The model under review builds one solid part; all positions refer to its coordinate system, in mm. Coordinates: 2 decimals unless noted, no trailing zeros. Order: outer loops, then holes, each group sorted by start corner. A loop starts at its lowest first (then second) coordinate and runs counter-clockwise, first axis right, second up. Notation, with made-up numbers: M -29,39 L 21,39 A28 ccw 21,72 Z; hole C 81.25,52 d6. An arc over 180 degrees is marked long. One line per item, written item: value.
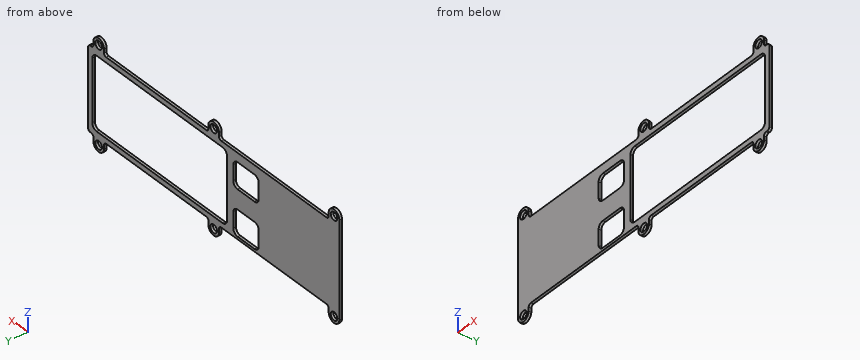
Autodesk Inventor part; units mm, degrees
ref_plane "YZ Plane" through (0, 0, 0) normal (1, 0, 0) x (0, 1, 0)
ref_plane "XZ Plane" through (0, 0, 0) normal (0, 1, 0) x (-1, 0, 0)
ref_plane "XY Plane" through (0, 0, 0) normal (0, 0, 1) x (1, 0, 0)
sketch "Sketch1" plane through (0, 0, 0) normal (0, 1, 0) x (-1, 0, 0)
  line L0 (0, 0) -> (37, 0) construction
  line L1 (37, 0) -> (37, -30) construction
  line L2 (37, -30) -> (0, -30) construction
  line L3 (0, -30) -> (0, 0) construction
  line L4 (75.5, -6) -> (38, -6) construction
  line L5 (38, -6) -> (38, -24) construction
  line L6 (38, -24) -> (75.5, -24) construction
  line L7 (75.5, -24) -> (75.5, -6) construction
  line L8 (94, 0) -> (76.5, 0) construction
  line L9 (76.5, 0) -> (76.5, -28) construction
  line L10 (76.5, -28) -> (94, -28) construction
  line L11 (94, -28) -> (94, 0) construction
  line L12 (-1, 1) -> (117.5, 1)
  line L13 (117.5, 1) -> (117.5, -31)
  line L14 (117.5, -31) -> (-1, -31)
  line L15 (-1, -31) -> (-1, 1)
  line L16 (0, 0) -> (94, 0)
  line L17 (94, 0) -> (94, -30)
  line L18 (94, -30) -> (0, -30)
  line L19 (0, -30) -> (0, 0)
  line L20 (38, -8) -> (37, -8)
  line L21 (37, -8) -> (37, -22)
  line L22 (37, -22) -> (38, -22)
  line L23 (38, -22) -> (38, -8)
  line L24 (73.5, -6) -> (40, -6)
  line L25 (40, -6) -> (40, -5)
  line L26 (40, -5) -> (73.5, -5)
  line L27 (73.5, -5) -> (73.5, -6)
  line L28 (73.5, -24) -> (40, -24)
  line L29 (40, -24) -> (40, -25)
  line L30 (40, -25) -> (73.5, -25)
  line L31 (73.5, -25) -> (73.5, -24)
  line L32 (76.5, -8) -> (75.5, -8)
  line L33 (75.5, -8) -> (75.5, -22)
  line L34 (75.5, -22) -> (76.5, -22)
  line L35 (76.5, -22) -> (76.5, -8)
  line L36 (115, -31) -> (115, -33.5) construction
  line L37 (58.25, -31) -> (58.25, -33.5) construction
  line L38 (4, -31) -> (4, -33.5) construction
  line L39 (115, 1) -> (115, 3.5) construction
  line L40 (58.25, 1) -> (58.25, 3.5) construction
  line L41 (4, 1) -> (4, 3.5) construction
  circle A0 centre (115, -33.5) radius 2.5
  circle A1 centre (58.25, -33.5) radius 2.5
  circle A2 centre (4, -33.5) radius 2.5
  circle A3 centre (4, 3.5) radius 2.5
  circle A4 centre (58.25, 3.5) radius 2.5
  circle A5 centre (115, 3.5) radius 2.5
  line L42 (117.5, 1) -> (117.5, 3.5)
  line L43 (112.5, 3.5) -> (112.5, 1)
  line L44 (60.75, 3.5) -> (60.75, 1)
  line L45 (55.75, 3.5) -> (55.75, 1)
  line L46 (6.5, 3.5) -> (6.5, 1)
  line L47 (1.5, 3.5) -> (1.5, 1)
  line L48 (1.5, -33.5) -> (1.5, -31)
  line L49 (6.5, -33.5) -> (6.5, -31)
  line L50 (55.75, -33.5) -> (55.75, -31)
  line L51 (60.75, -33.5) -> (60.75, -31)
  line L52 (117.5, -33.5) -> (117.5, -31)
  line L53 (112.5, -33.5) -> (112.5, -31)
  circle A6 centre (115, -33.5) radius 1.55
  circle A7 centre (58.25, -33.5) radius 1.55
  circle A8 centre (4, -33.5) radius 1.55
  circle A9 centre (4, 3.5) radius 1.55
  circle A10 centre (58.25, 3.5) radius 1.55
  circle A11 centre (115, 3.5) radius 1.55
  line L54 (57.75, -30) -> (58.75, -30)
  line L55 (58.75, -30) -> (58.75, -25)
  line L56 (58.75, -25) -> (57.75, -25)
  line L57 (57.75, -25) -> (57.75, -30)
  line L58 (57.75, -5) -> (58.75, -5)
  line L59 (58.75, -5) -> (58.75, 0)
  line L60 (58.75, 0) -> (57.75, 0)
  line L61 (57.75, 0) -> (57.75, -5)
  line L62 (40, -25) -> (41, -25)
  line L63 (41, -25) -> (41, -30)
  line L64 (41, -30) -> (40, -30)
  line L65 (40, -30) -> (40, -25)
  line L66 (40, -5) -> (41, -5)
  line L67 (41, -5) -> (41, 0)
  line L68 (41, 0) -> (40, 0)
  line L69 (40, 0) -> (40, -5)
  line L70 (73.5, -5) -> (72.5, -5)
  line L71 (72.5, -5) -> (72.5, 0)
  line L72 (72.5, 0) -> (73.5, 0)
  line L73 (73.5, 0) -> (73.5, -5)
  line L74 (73.5, -25) -> (72.5, -25)
  line L75 (72.5, -25) -> (72.5, -30)
  line L76 (72.5, -30) -> (73.5, -30)
  line L77 (73.5, -30) -> (73.5, -25)
  dimension "d0" = 37
  dimension "d1" = 30
  dimension "d2" = 18
  dimension "d3" = 37.5
  dimension "d4" = 1
  dimension "d5" = 6
  dimension "d6" = 17.5
  dimension "d7" = 28
  dimension "d8" = 1
  dimension "d9" = 1
  dimension "d10" = 1
  dimension "d11" = 1
  dimension "d12" = 117.5
  dimension "d13" = 2
  dimension "d14" = 2
  dimension "d15" = 1
  dimension "d16" = 1
  dimension "d17" = 2
  dimension "d18" = 2
  dimension "d19" = 2
  dimension "d20" = 2
  dimension "d21" = 2.5
  dimension "d22" = 2.5
  dimension "d23" = 5
  dimension "d24" = 2.5
  dimension "d25" = 2.5
  dimension "d26" = 2.5
  dimension "d27" = 2.5
  dimension "d28" = 5
  dimension "d29" = 5
  dimension "d30" = 2.5
  dimension "d31" = 3.1
  dimension "d32" = 3.1
  dimension "d33" = 3.1
  dimension "d34" = 3.1
  dimension "d35" = 3.1
  dimension "d36" = 3.1
  dimension "d44" = 1
  dimension "d45" = 1
  dimension "d46" = 0.5
  dimension "d47" = 0
  dimension "d48" = 1
  dimension "d49" = 1
  dimension "d50" = 1
  dimension "d51" = 1
extrude "Extrusion1" add sketch "Sketch1" along normal blind 7 contours L12 L13 L14 L15 | L47 A3 L12 | A3 L46 L12 | A3 | L14 A2 L48 | L14 L49 A2 | A2 | L45 A4 L12 | A4 L44 L12 | A4 | L14 A1 L50 | L14 L51 A1 | A1 | L43 A5 L12 | A5 L42 L12 | A5 | L14 A0 L53 | L14 L52 A0 | A0 | L16 L67 L26 L69 | L26 L27 L24 L25 | L65 L30 L63 L18 | L16 L59 L26 L61 | L29 L28 L31 L30 | L57 L30 L55 L18 | L16 L73 L26 L71 | L75 L30 L77 L18 | L23 L22 L21 L20 | L35 L34 L33 L32
sketch "Sketch2" plane through (0, 0, 0) normal (0, -1, 0) x (1, 0, 0)
  line L0 (-117.5, -33.5) -> (-117.5, 3.5)
  arc A0 (-117.5, -33.5) -> (-112.5, -33.5) centre (-115, -33.5) ccw
  line L1 (-112.5, -31) -> (-112.5, -33.5)
  line L2 (-60.75, -31) -> (-112.5, -31)
  line L3 (-60.75, -33.5) -> (-60.75, -31)
  arc A1 (-60.75, -33.5) -> (-55.75, -33.5) centre (-58.25, -33.5) ccw
  line L4 (-55.75, -31) -> (-55.75, -33.5)
  line L5 (-6.5, -31) -> (-55.75, -31)
  line L6 (-6.5, -33.5) -> (-6.5, -31)
  arc A2 (-6.5, -33.5) -> (-1.5, -33.5) centre (-4, -33.5) ccw
  line L7 (-1.5, -31) -> (-1.5, -33.5)
  line L8 (1, -31) -> (-1.5, -31)
  line L9 (1, 1) -> (1, -31)
  line L10 (-1.5, 1) -> (1, 1)
  line L11 (-1.5, 3.5) -> (-1.5, 1)
  arc A3 (-1.5, 3.5) -> (-6.5, 3.5) centre (-4, 3.5) ccw
  line L12 (-6.5, 1) -> (-6.5, 3.5)
  line L13 (-55.75, 1) -> (-6.5, 1)
  line L14 (-55.75, 3.5) -> (-55.75, 1)
  arc A4 (-55.75, 3.5) -> (-60.75, 3.5) centre (-58.25, 3.5) ccw
  line L15 (-60.75, 1) -> (-60.75, 3.5)
  line L16 (-112.5, 1) -> (-60.75, 1)
  line L17 (-112.5, 3.5) -> (-112.5, 1)
  arc A5 (-112.5, 3.5) -> (-117.5, 3.5) centre (-115, 3.5) ccw
  circle A6 centre (-58.25, 3.5) radius 1.55
  circle A7 centre (-4, 3.5) radius 1.55
  circle A8 centre (-4, -33.5) radius 1.55
  circle A9 centre (-58.25, -33.5) radius 1.55
  circle A10 centre (-115, 3.5) radius 1.55
  circle A11 centre (-115, -33.5) radius 1.55
  line L18 (-41, 0) -> (-57.75, 0)
  line L19 (0, -30) -> (0, 0)
  line L20 (-57.75, -30) -> (-41, -30)
  line L21 (-94, 0) -> (-94, -30)
  line L22 (-41, -5) -> (-41, 0)
  line L23 (-57.75, -5) -> (-41, -5)
  line L24 (-57.75, 0) -> (-57.75, -5)
  line L25 (-41, -30) -> (-41, -25)
  line L26 (-57.75, -25) -> (-57.75, -30)
  line L27 (-41, -25) -> (-57.75, -25)
  line L28 (-72.5, -25) -> (-72.5, -30)
  line L29 (-58.75, -25) -> (-72.5, -25)
  line L30 (-58.75, -30) -> (-58.75, -25)
  line L31 (-72.5, -30) -> (-58.75, -30)
  line L32 (-72.5, 0) -> (-72.5, -5)
  line L33 (-58.75, 0) -> (-72.5, 0)
  line L34 (-58.75, -5) -> (-58.75, 0)
  line L35 (-72.5, -5) -> (-58.75, -5)
  line L36 (-73.5, 0) -> (-94, 0)
  line L37 (-73.5, -6) -> (-73.5, 0)
  line L38 (-40, -6) -> (-73.5, -6)
  line L39 (-40, 0) -> (-40, -6)
  line L40 (0, 0) -> (-40, 0)
  line L41 (-40, -30) -> (0, -30)
  line L42 (-40, -24) -> (-40, -30)
  line L43 (-73.5, -24) -> (-40, -24)
  line L44 (-73.5, -30) -> (-73.5, -24)
  line L45 (-94, -30) -> (-73.5, -30)
extrude "Extrusion2" add sketch "Sketch2" along normal blind 1 contours L0 A5 L17 L16 L15 A4 L14 L13 L12 A3 L11 L10 L9 L8 L7 A2 L6 L5 L4 A1 L3 L2 L1 A0 | L22 L23 L24 L18 | L41 L42 L43 L44 L45 L21 L36 L37 L38 L39 L40 L19 | L26 L27 L25 L20 | L29 L30 L31 L28 | L33 L34 L35 L32
fillet "Fillet2" radius 1 32 edges at (-73.5, 3.5, -6) (-73.5, 3.5, -24) (-40, 3.5, -24) (1, 3, -31) (-1.5, 3, -31) (1, 3, 1) (-55.75, 3, -31) (-1.5, 3, 1) (-55.75, 3, 1) (-112.5, 3, 1) (-112.5, 3, -31) (-60.75, 3, -31) (-6.5, 3, -31) (-60.75, 3, 1) (-6.5, 3, 1) (-40, 3.5, -6) (-72.5, 3.5, 0) (-57.75, 3.5, 0) (-72.5, 3.5, -25) (-57.75, 3.5, -25) (-41, 3.5, -25) (-58.75, 3.5, -25) (-41, 3.5, 0) (-58.75, 3.5, 0) (-72.5, 3.5, -30) (-57.75, 3.5, -30) (-57.75, 3.5, -5) (-72.5, 3.5, -5) (-41, 3.5, -5) (-58.75, 3.5, -5) (-58.75, 3.5, -30) (-41, 3.5, -30)
sketch "Sketch5" plane through (0, 7, 0) normal (0, 1, 0) x (1, 0, 0)
  line L0 (-120.447, 38.9055) -> (3.6698, 38.9055)
  line L1 (3.6698, 38.9055) -> (3.6698, -10.7705)
  line L2 (3.6698, -10.7705) -> (-120.447, -10.7705)
  line L3 (-120.447, -10.7705) -> (-120.447, 38.9055)
  point P0 (0, 0)
extrude "Extrusion5" cut sketch "Sketch5" against normal blind 7
sketch "Sketch13" plane through (0, 0, 0) normal (0, 1, 0) x (1, 0, 0)
  line L0 (-64.5, 29) -> (-1, 29)
  line L1 (-1, 29) -> (-1, 1)
  line L2 (-1, 1) -> (-64.5, 1)
  line L3 (-64.5, 1) -> (-64.5, 29)
  line L4 (1, 30) -> (1, 0)
  line L5 (-54.75, 31) -> (-7.5, 31)
  line L6 (-7.5, -1) -> (-54.75, -1)
  line L7 (-117.5, -3.5) -> (-117.5, 33.5)
  line L8 (-79.5, 30) -> (-67.5, 30)
  line L9 (-67.5, 30) -> (-67.5, 20)
  line L10 (-67.5, 20) -> (-79.5, 20)
  line L11 (-79.5, 20) -> (-79.5, 30)
  line L12 (-79.5, 12.5) -> (-67.5, 12.5)
  line L13 (-67.5, 12.5) -> (-67.5, 2.5)
  line L14 (-67.5, 2.5) -> (-79.5, 2.5)
  line L15 (-79.5, 2.5) -> (-79.5, 12.5)
  line L16 (-111.5, 31) -> (-61.75, 31)
  line L17 (-61.75, -1) -> (-111.5, -1)
  line L18 (-76.1794, 28.5) -> (-69.1572, 28.5) construction
  line L19 (-69.1572, 28.5) -> (-69.1572, 21.5) construction
  line L20 (-69.1572, 21.5) -> (-76.1794, 21.5) construction
  line L21 (-76.1794, 21.5) -> (-76.1794, 28.5) construction
  point P0 (0, 0)
  point P1 (-79.5, 25)
  point P2 (-79.5, 7.5)
  point P3 (-67.5, 25)
  point P4 (-67.5, 7.5)
  dimension "d114" = 2
  dimension "d115" = 2
  dimension "d116" = 2
  dimension "d117" = 53
  dimension "d118" = 50
  dimension "d119" = 12
  dimension "d120" = 1
  dimension "d121" = 3.5
  dimension "d122" = 13.5
  dimension "d123" = 11
  dimension "d127" = 2.5
  dimension "d128" = 9.5
extrude "Extrusion15" cut sketch "Sketch13" against normal through all
fillet "Fillet4" radius 2 12 edges at (-64.5, -0.5, -29) (-79.5, -0.5, -30) (-79.5, -0.5, -12.5) (-1, -0.5, -29) (-1, -0.5, -1) (-67.5, -0.5, -2.5) (-67.5, -0.5, -20) (-64.5, -0.5, -1) (-79.5, -0.5, -2.5) (-79.5, -0.5, -20) (-67.5, -0.5, -30) (-67.5, -0.5, -12.5)
properties part number "frontpackCOVER1"
(1) For L1, parallel to Z at x = -115, y = -0.4; L2, parallel to X at y = -0.85, z = -23; L3, parallel to Z at x = -4, y = -0.35, list the stretches that pass through material, from the lowest coordinate up.
Geometry results:
L1: z = -36 to -35.05, -31.95 to 1.95, 5.05 to 6
L2: x = -117.5 to -79.5, -67.5 to -64.5, -1 to 1
L3: z = -36 to -35.05, -31.95 to -29, -1 to 1.95, 5.05 to 6
(2) We need section A-A, the plane x = -115. State the section outline as (y, z) points.
Geometry results:
outline: M -1,-36 L 0,-36 L 0,-35.05 L -1,-35.05 Z; M -1,-31.95 L 0,-31.95 L 0,1.95 L -1,1.95 Z; M -1,5.05 L 0,5.05 L 0,6 L -1,6 Z
(3) We need section C-C, the plane x = -58.25. State the section outline as (y, z) points, plus the area to 3 significant figures.
Geometry results:
outline: M -1,-36 L 0,-36 L 0,-35.05 L -1,-35.05 Z; M -1,-31.95 L 0,-31.95 L 0,-29 L -1,-29 Z; M -1,-1 L 0,-1 L 0,1.95 L -1,1.95 Z; M -1,5.05 L 0,5.05 L 0,6 L -1,6 Z
area: 7.80 mm2
(4) We need section B-B, the plane z = -25. State the section outline as (x, y) points.
Geometry results:
outline: M -117.5,-1 L -79.5,-1 L -79.5,0 L -117.5,0 Z; M -67.5,-1 L -64.5,-1 L -64.5,0 L -67.5,0 Z; M -1,-1 L 1,-1 L 1,0 L -1,0 Z
(5) Insertion check: pin 1 Ø0.5 at (x, y) = (-72, -0.5) entering from -Z; pin 2 Ø1.9 at (x, z) = (-115, 3.5) entering from +Y. Each pin has a flat end and moves straight along its axis. Give the tip position at first contact, or say it passes through.
Geometry results:
pin 1: stops at z = -31
pin 2: passes through
(6) We need section D-D, the plane x = -19.5. State the section outline as (y, z) points, plus the area to 3 significant figures.
Geometry results:
outline: M -1,-31 L 0,-31 L 0,-29 L -1,-29 Z; M -1,-1 L 0,-1 L 0,1 L -1,1 Z
area: 4.00 mm2
